from build123d import *

# Parameters (mm, degrees)
BOSS_EXTRUDE1_DEPTH      = 10
BOSS_EXTRUDE1_DEPTH_BACK = 26
SKETCH1_W                = 40.4
SKETCH1_H                = 19.8
SKETCH2_W                = 7.1
SKETCH2_H                = 19.8
SKETCH2_R                = 2.1
BOSS_EXTRUDE2_DEPTH      = 2.5
SKETCH3_W                = 7.1
SKETCH3_H                = 19.8
SKETCH3_R                = 2.1
BOSS_EXTRUDE3_DEPTH      = 2.5
BOSS_EXTRUDE4_START      = 10
SKETCH4_R                = 6
BOSS_EXTRUDE4_DEPTH      = 2
BOSS_EXTRUDE5_START      = 12
SKETCH5_R                = 3
BOSS_EXTRUDE5_DEPTH      = 2


with BuildPart() as part:
    # Sketch1 → Boss-Extrude1 (new, two sides: drawn at the far end of the back side and taken through both)
    with BuildSketch(Plane.XY.offset(-BOSS_EXTRUDE1_DEPTH_BACK)):
        with Locations((10.2, 0)):
            Rectangle(SKETCH1_W, SKETCH1_H)
    extrude(amount=BOSS_EXTRUDE1_DEPTH + BOSS_EXTRUDE1_DEPTH_BACK)

    # Sketch2 → Boss-Extrude2 (add)
    with BuildSketch(Plane.XY):
        with Locations((-13.55, 0)):
            Rectangle(SKETCH2_W, SKETCH2_H)
        with Locations((-13.8, 5)):
            Circle(SKETCH2_R, mode=Mode.SUBTRACT)
        with Locations((-13.8, -5)):
            Circle(SKETCH2_R, mode=Mode.SUBTRACT)
    extrude(amount=BOSS_EXTRUDE2_DEPTH)

    # Sketch3 → Boss-Extrude3 (add)
    with BuildSketch(Plane.XY):
        with Locations((33.95, 0)):
            Rectangle(SKETCH3_W, SKETCH3_H)
        with Locations((34.2, 5)):
            Circle(SKETCH3_R, mode=Mode.SUBTRACT)
        with Locations((34.2, -5)):
            Circle(SKETCH3_R, mode=Mode.SUBTRACT)
    extrude(amount=BOSS_EXTRUDE3_DEPTH)

    # Sketch4 → Boss-Extrude4 (add)
    with BuildSketch(Plane.XY.offset(BOSS_EXTRUDE4_START)):
        Circle(SKETCH4_R)
    extrude(amount=BOSS_EXTRUDE4_DEPTH)

    # Sketch5 → Boss-Extrude5 (add)
    with BuildSketch(Plane.XY.offset(BOSS_EXTRUDE5_START)):
        Circle(SKETCH5_R)
    extrude(amount=BOSS_EXTRUDE5_DEPTH)


solid = part.part
For this review, take the finished solid that the model builds, in its own axes (mm). A direction names the side the tool comes from. Round coordinates to 2 decimals unless told otherwise and drop trailing zeros. Order: outer loops, then holes, each group sorted by start corner. A loop starts at its lowest first (then second) coordinate and runs counter-clockwise, first axis right, second up. Notation, with made-up numbers: M -37.75,3 L -20.75,3 A24 ccw -20.75,22 Z; hole C -5.5,8 d4. An arc over 180 degrees is marked long. Use a Markdown table: item, result. Add a question column.
Item 1: Add section A-A, the plane x = 34.2. Give the boundary of the cut face in (y, z).
Item 2: Add section D-D, the plane y = -8.5. Give the boundary of the cut face in (x, z).
Item 3: Mouldability with a two-part tool opening along Y and no side actions: class faces 1 (the flat face through (0, 0, 14)), 2 (the cylindrical face through (32.1, -4.91, 1.23)), 3 (the flat face through (10, 9.9, -8)) as released by +Y, released by -Y, zero draft, split by the parting line, or undercut.
Item 4: Tool access review of faces 4 (the cylindrical face through (-6, 0, 11)), 5 (the flat face through (-10, 0, -13)), 6 (the flat face through (30.4, 0, 6)), 7 (the flat face through (30.4, 0, -13)): name each direction out of +Z, -Z, +X, -X, +Y, -Y from which nothing blocks a thin tool from reaching the whole face with its end or side.
Item 5: Insertion check: pin 1 (6 mm diameter, centred on y = -4.5, z = 8, fed in from -X); pin 2 (3 mm diameter, centred on x = -5.5, y = 4.5, fed in from +Z); pin 3 (10 mm diameter, centred on y = -4.5, z = -14.5, fed in from +X); pin 4 (2 mm diameter, centred on x = 34.5, y = -4, fed in from -Z). Each pin has a flat end and moves straight along its axis. Give the tip position at first contact, or say it passes through.
Item 6: To check wall thickness, follow line 1 along Y through (x, z) = (34.2, 0.9); line 2 along Z through (x, y) = (30, 2.5); line 3 along Y through (x, z) = (-13, 1). State the ranges of each line that lie inside material, in increasing order.
Item 7: Add section B-B, the plane y = 0. Give the boundary of the cut face in (x, z), then the cut area to 3 significant figures.
Item 8: Add section C-C, the plane y = -4. Give the boundary of the cut face in (x, z).
Geometry results:
| question | item | result |
|---|---|---|
| 1 | outline | M -9.9,0 L -7.1,0 L -7.1,2.5 L -9.9,2.5 Z; M -2.9,0 L 2.9,0 L 2.9,2.5 L -2.9,2.5 Z; M 7.1,0 L 9.9,0 L 9.9,2.5 L 7.1,2.5 Z |
| 2 | outline | M -17.1,0 L -10,0 L -10,-26 L 30.4,-26 L 30.4,0 L 37.5,0 L 37.5,2.5 L 30.4,2.5 L 30.4,10 L -10,10 L -10,2.5 L -17.1,2.5 Z |
| 3 | face 1 | zero draft |
| 3 | face 2 | undercut |
| 3 | face 3 | released by +Y |
| 4 | face 4 | +Z |
| 4 | face 5 | -Z, -X, +Y, -Y |
| 4 | face 6 | +Z, +X, +Y, -Y |
| 4 | face 7 | -Z, +X, +Y, -Y |
| 5 | pin 1 | stops at x = -10 |
| 5 | pin 2 | stops at z = 12 |
| 5 | pin 3 | stops at x = 30.4 |
| 5 | pin 4 | passes through |
| 6 | line 1 | y = -9.9 to -7.1, -2.9 to 2.9, 7.1 to 9.9 |
| 6 | line 2 | z = -26 to 10 |
| 6 | line 3 | y = -9.9 to -6.94, -3.06 to 3.06, 6.94 to 9.9 |
| 7 | outline | M -17.1,0 L -10,0 L -10,-26 L 30.4,-26 L 30.4,0 L 37.5,0 L 37.5,2.5 L 30.4,2.5 L 30.4,10 L 6,10 L 6,12 L 3,12 L 3,14 L -3,14 L -3,12 L -6,12 L -6,10 L -10,10 L -10,2.5 L -17.1,2.5 Z |
| 7 | area | 1,530 mm² |
| 8 | outline | M -17.1,0 L -15.65,0 L -15.65,2.5 L -17.1,2.5 Z; M -11.95,0 L -10,0 L -10,-26 L 30.4,-26 L 30.4,0 L 32.35,0 L 32.35,2.5 L 30.4,2.5 L 30.4,10 L 4.47,10 L 4.47,12 L -4.47,12 L -4.47,10 L -10,10 L -10,2.5 L -11.95,2.5 Z; M 36.05,0 L 37.5,0 L 37.5,2.5 L 36.05,2.5 Z |
